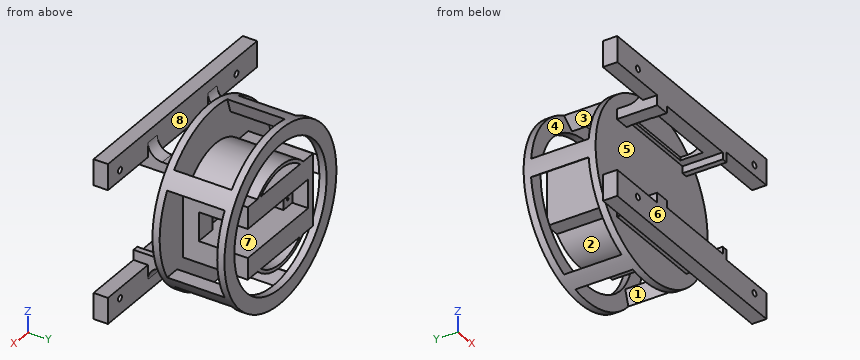
```python
from build123d import *

# Parameters (mm, degrees)
ESQUISSE1_W                  = 70
ESQUISSE1_H                  = 50
BOSS_EXTRU_1_DEPTH           = 50
ESQUISSE2_W                  = 40.5
ESQUISSE2_H                  = 20
ENL_V_MAT_EXTRU_1_DEPTH      = 38
ESQUISSE3_W                  = 9.502474521
ESQUISSE3_H                  = 20
ENL_V_MAT_EXTRU_2_DEPTH      = 11
ESQUISSE4_R                  = 60.076490873
ESQUISSE4_R_2                = 49.5
BOSS_EXTRU_2_DEPTH           = 50
ESQUISSE5_W                  = 60
ESQUISSE5_H                  = 40
ENL_V_MAT_EXTRU_3_DEPTH      = 24
R_P_TITION_START             = -20
R_P_TITION_CIRCULAIRE1_DEPTH = 40
ESQUISSE12_W                 = 74.3
ESQUISSE12_H                 = 74.3
BOSS_EXTRU_7_DEPTH           = 28
ESQUISSE13_W                 = 160
ESQUISSE13_H                 = 18
BOSS_EXTRU_8_DEPTH           = 10
ESQUISSE15_R                 = 60.076490873
BOSS_EXTRU_9_DEPTH           = 5
ESQUISSE16_W                 = 60
ESQUISSE16_H                 = 70
ENL_V_MAT_EXTRU_4_DEPTH      = 28
ENL_V_MAT_EXTRU_5_REACH      = 156.276
ESQUISSE17_W                 = 60.3
ESQUISSE17_H                 = 28
ENL_V_MAT_EXTRU_6_REACH      = 138.609
ESQUISSE18_W                 = 54.3
ESQUISSE18_H                 = 15.510808694
TROU_TARAUD_M5X0_82_D        = 4.2
TROU_TARAUD_M5X0_82_DEPTH    = 54.927
TROU_TARAUD_M5X0_82_TIP      = 1.2618073
TROU_TARAUD_M5X0_83_D        = 4.2
TROU_TARAUD_M5X0_83_DEPTH    = 54.927
TROU_TARAUD_M5X0_83_TIP      = 1.2618073
CONG_1_R                     = 10
ESQUISSE25_W                 = 16.470730929
ESQUISSE25_H                 = 20
ENL_V_MAT_EXTRU_7_DEPTH      = 34
TROU_TARAUD_M2X0_41_D        = 1.6
TROU_TARAUD_M2X0_41_DEPTH    = 15
TROU_TARAUD_M2X0_41_TIP      = 0.480688495


# Read off the part's stored shape, not the designer's step: Répétition circulaire1
with BuildPart() as part:
    # Esquisse1 → Boss.-Extru.1 (new body)
    with BuildSketch(Plane.XY):
        Rectangle(ESQUISSE1_W, ESQUISSE1_H)
    extrude(amount=BOSS_EXTRU_1_DEPTH)

    # Esquisse2 → Enlèv. mat.-Extru.1 (cut)
    with BuildSketch(Plane(origin=(0, 25, 0), x_dir=(1, 0, 0), z_dir=(0, 1, 0))):
        with Locations((0, -25)):
            Rectangle(ESQUISSE2_W, ESQUISSE2_H)
    extrude(amount=-ENL_V_MAT_EXTRU_1_DEPTH, mode=Mode.SUBTRACT)

    # Esquisse3 → Enlèv. mat.-Extru.2 (cut)
    with BuildSketch(Plane(origin=(0, 25, 0), x_dir=(1, 0, 0), z_dir=(0, 1, 0))):
        with Locations((25.001237261, -25)):
            Rectangle(ESQUISSE3_W, ESQUISSE3_H)
        with Locations((-25.001237261, -25)):
            Rectangle(ESQUISSE3_W, ESQUISSE3_H)
    extrude(amount=-ENL_V_MAT_EXTRU_2_DEPTH, mode=Mode.SUBTRACT)

    # Esquisse4 → Boss.-Extru.2 (add)
    # profile 1 of 7: a face of its own
    with BuildSketch(Plane(origin=(0, 25, 0), x_dir=(1, 0, 0), z_dir=(0, 1, 0))):
        with Locations(Location((0, -25.176679726, 0), (0, 0, 270))):
            Circle(ESQUISSE4_R)
        with Locations(Location((0, -25.176679726, 0), (0, 0, 270))):
            Circle(ESQUISSE4_R_2, mode=Mode.SUBTRACT)
    # profile 2 of 7: a face of its own
    with BuildSketch(Plane(origin=(0, 25, 0), x_dir=(1, 0, 0), z_dir=(0, 1, 0))):
        with BuildLine():
            ThreePointArc((24.673928965, -50), (32.315534297, -38.619381951), (35, -25.176679726))
            ThreePointArc((35, -25.176679726), (32.217729855, -11.501231543), (24.313263828, 0))
            Line((24.313263828, 0), (20.744399349, 0))
            ThreePointArc((20.744399349, 0), (29.503552635, -11.257782921), (32.622006474, -25.176679726))
            ThreePointArc((32.622006474, -25.176679726), (29.619854452, -38.846336948), (21.16596506, -50))
            Line((21.16596506, -50), (24.673928965, -50))
        make_face()
    # profile 3 of 7: a face of its own
    with BuildSketch(Plane(origin=(0, 25, 0), x_dir=(1, 0, 0), z_dir=(0, 1, 0))):
        with BuildLine():
            Line((-20.744399349, 0), (-24.313263828, 0))
            ThreePointArc((-24.313263828, 0), (-34.99908948, -24.924220698), (-24.673928965, -50))
            Line((-24.673928965, -50), (-21.16596506, -50))
            ThreePointArc((-21.16596506, -50), (-32.620847034, -24.901643114), (-20.744399349, 0))
        make_face()
    # profile 4 of 7: a face of its own
    with BuildSketch(Plane(origin=(0, 25, 0), x_dir=(1, 0, 0), z_dir=(0, 1, 0))):
        with BuildLine():
            Line((20.744399349, 0), (24.313263828, 0))
            ThreePointArc((24.313263828, 0), (0, 9.823320274), (-24.313263828, 0))
            Line((-24.313263828, 0), (-20.744399349, 0))
            ThreePointArc((-20.744399349, 0), (0, 7.445326748), (20.744399349, 0))
        make_face()
    # profile 5 of 7: a face of its own
    with BuildSketch(Plane(origin=(0, 25, 0), x_dir=(1, 0, 0), z_dir=(0, 1, 0))):
        with BuildLine():
            ThreePointArc((24.673928965, -50), (32.315534297, -38.619381951), (35, -25.176679726))
            ThreePointArc((35, -25.176679726), (32.217729855, -11.501231543), (24.313263828, 0))
            Line((24.313263828, 0), (20.744399349, 0))
            ThreePointArc((20.744399349, 0), (29.503552635, -11.257782921), (32.622006474, -25.176679726))
            ThreePointArc((32.622006474, -25.176679726), (29.619854452, -38.846336948), (21.16596506, -50))
            Line((21.16596506, -50), (24.673928965, -50))
        make_face()
    # profile 6 of 7: a face of its own
    with BuildSketch(Plane(origin=(0, 25, 0), x_dir=(1, 0, 0), z_dir=(0, 1, 0))):
        with BuildLine():
            Line((-20.744399349, 0), (-24.313263828, 0))
            ThreePointArc((-24.313263828, 0), (-34.99908948, -24.924220698), (-24.673928965, -50))
            Line((-24.673928965, -50), (-21.16596506, -50))
            ThreePointArc((-21.16596506, -50), (-32.620847034, -24.901643114), (-20.744399349, 0))
        make_face()
    # profile 7 of 7: a face of its own
    with BuildSketch(Plane(origin=(0, 25, 0), x_dir=(1, 0, 0), z_dir=(0, 1, 0))):
        with BuildLine():
            ThreePointArc((-24.673928965, -50), (0, -60.176679726), (24.673928965, -50))
            Line((24.673928965, -50), (21.16596506, -50))
            ThreePointArc((21.16596506, -50), (0, -57.798686199), (-21.16596506, -50))
            Line((-21.16596506, -50), (-24.673928965, -50))
        make_face()
    extrude(amount=-BOSS_EXTRU_2_DEPTH)


with BuildPart() as boss_extru_2_piece_1:
    # of the separate pieces the step leaves, piece 1, a body of its own (boss_extru_2_pieces)
    add(part.part.solids().sort_by_distance((0, 25, 85.253170599))[0])

    # Esquisse5 → Enlèv. mat.-Extru.3 (cut)
    with BuildSketch(Plane(origin=(60.076490873, 0, 0), x_dir=(0, 0, -1), z_dir=(1, 0, 0))):
        with Locations((-25.176679726, 0)):
            Rectangle(ESQUISSE5_W, ESQUISSE5_H)
    extrude(amount=-ENL_V_MAT_EXTRU_3_DEPTH, mode=Mode.SUBTRACT)

    # Répétition circulaire1 outline → Répétition circulaire1 (cut)
    with BuildSketch(Plane(origin=(0, 0, 0), x_dir=(1, 0, 0), z_dir=(0, 1, 0)).offset(R_P_TITION_START)):
        with BuildLine():
            Line((39.373214245, 4.823320274), (41.291457614, 4.823320274))
            Line((41.291457614, 4.823320274), (44.615977372, 15.055140003))
            ThreePointArc((44.615977372, 15.055140003), (18.564656642, 31.959458395), (-12.447413605, 33.596159666))
            Line((-12.447413605, 33.596159666), (-15.771933364, 23.364339937))
            Line((-15.771933364, 23.364339937), (-24.475639087, 29.687952296))
            ThreePointArc((-24.475639087, 29.687952296), (-48.602902078, 10.135395619), (-59.742754225, -18.853067366))
            Line((-59.742754225, -18.853067366), (-51.039048501, -25.176679726))
            Line((-51.039048501, -25.176679726), (-59.742754225, -31.500292085))
            ThreePointArc((-59.742754225, -31.500292085), (-48.602902079, -60.488755071), (-24.475639087, -80.041311748))
            Line((-24.475639087, -80.041311748), (-15.771933364, -73.717699388))
            Line((-15.771933364, -73.717699388), (-12.447413605, -83.949519118))
            ThreePointArc((-12.447413605, -83.949519118), (18.564656643, -82.312817847), (44.615977373, -65.408499455))
            Line((44.615977373, -65.408499455), (41.291457614, -55.176679726))
            Line((41.291457614, -55.176679726), (39.373214245, -55.176679726))
            ThreePointArc((39.373214245, -55.176679726), (-49.5, -25.176679726), (39.373214245, 4.823320274))
        make_face()
    extrude(amount=R_P_TITION_CIRCULAIRE1_DEPTH, mode=Mode.SUBTRACT)



with BuildPart() as boss_extru_2_piece_2:
    # of the separate pieces the step leaves, piece 2, a body of its own (boss_extru_2_pieces)
    add(part.part.solids().sort_by_distance((-35, 25, 0))[0])


with BuildPart() as boss_extru_2_piece_1_1:
    add(boss_extru_2_piece_1.part)

    add(boss_extru_2_piece_2.part)  # Boss.-Extru.7 merges Boss.-Extru.2 piece 2
    # Esquisse12 → Boss.-Extru.7 (add)
    with BuildSketch(Plane.XZ.offset(25)):
        with Locations((0, 25.176679726)):
            Rectangle(ESQUISSE12_W, ESQUISSE12_H)
    extrude(amount=BOSS_EXTRU_7_DEPTH)

    # Esquisse13 → Boss.-Extru.8 (add)
    with BuildSketch(Plane.XZ.offset(53)):
        with Locations((0, 71.326679726)):
            Rectangle(ESQUISSE13_W, ESQUISSE13_H)
        with Locations((0, -20.973320274)):
            Rectangle(ESQUISSE13_W, ESQUISSE13_H)
    extrude(amount=-BOSS_EXTRU_8_DEPTH)

    # Esquisse15 → Boss.-Extru.9 (add)
    with BuildSketch(Plane(origin=(0, -20, 0), x_dir=(1, 0, 0), z_dir=(0, 1, 0))):
        with Locations(Location((0, -25.176679726, 0), (0, 0, 270))):
            Circle(ESQUISSE15_R)
    extrude(amount=-BOSS_EXTRU_9_DEPTH)

    # Esquisse16 → Enlèv. mat.-Extru.4 (cut)
    with BuildSketch(Plane.XZ.offset(53)):
        with Locations((3.15, 25.176679726)):
            Rectangle(ESQUISSE16_W, ESQUISSE16_H)
    extrude(amount=-ENL_V_MAT_EXTRU_4_DEPTH, mode=Mode.SUBTRACT)

    # Enlèv. mat.-Extru.5: up to this face of the body (flat: up to its plane)
    enl_v_mat_extru_5_end = Plane(boss_extru_2_piece_1_1.part.faces().sort_by_distance((-37.15, -39, 25.176679726))[0])
    # Esquisse17 → Enlèv. mat.-Extru.5 (cut, up to the picked face)
    with BuildSketch(Plane(origin=(37.15, 0, 0), x_dir=(0, 0, -1), z_dir=(1, 0, 0)), mode=Mode.PRIVATE) as enl_v_mat_extru_5_sk1:
        with Locations((-25.176679726, -39)):
            Rectangle(ESQUISSE17_W, ESQUISSE17_H)
    enl_v_mat_extru_5_tool1 = split(extrude(enl_v_mat_extru_5_sk1.sketch, amount=-ENL_V_MAT_EXTRU_5_REACH, mode=Mode.PRIVATE), bisect_by=enl_v_mat_extru_5_end, keep=Keep.BOTH, mode=Mode.PRIVATE)
    add(enl_v_mat_extru_5_tool1.solids().sort_by(Axis((37.15, -39, 25.17668), (-1, 0, 0)))[0], mode=Mode.SUBTRACT)

    # Enlèv. mat.-Extru.6: up to this face of the body (flat: up to its plane)
    enl_v_mat_extru_6_end = Plane(boss_extru_2_piece_1_1.part.faces().sort_by_distance((0, -34, -11.973320274))[0])
    # Esquisse18 → Enlèv. mat.-Extru.6 (cut, up to the picked face)
    with BuildSketch(Plane.XY.offset(62.326679726), mode=Mode.PRIVATE) as enl_v_mat_extru_6_sk1:
        with Locations((0, -35.244595653)):
            Rectangle(ESQUISSE18_W, ESQUISSE18_H)
    enl_v_mat_extru_6_tool1 = split(extrude(enl_v_mat_extru_6_sk1.sketch, amount=-ENL_V_MAT_EXTRU_6_REACH, mode=Mode.PRIVATE), bisect_by=enl_v_mat_extru_6_end, keep=Keep.BOTH, mode=Mode.PRIVATE)
    add(enl_v_mat_extru_6_tool1.solids().sort_by(Axis((0, -35.244596, 62.32668), (0, 0, -1)))[0], mode=Mode.SUBTRACT)

    # Trou taraudé M5x0.82
    with Locations(Plane(origin=(-57.931903984, -53, -18.999181229), x_dir=(0, 0, -1), z_dir=(0, -1, 0))):
        with Locations((0, 0), (-88.38422, 0.087735642)):
            Hole(TROU_TARAUD_M5X0_82_D / 2, depth=TROU_TARAUD_M5X0_82_DEPTH)
            with Locations((0, 0, -(TROU_TARAUD_M5X0_82_DEPTH + TROU_TARAUD_M5X0_82_TIP / 2))):  # 118° drill point
                Cone(0, TROU_TARAUD_M5X0_82_D / 2, TROU_TARAUD_M5X0_82_TIP, mode=Mode.SUBTRACT)

    # Trou taraudé M5x0.83
    with Locations(Plane(origin=(67.121659864, -53, 69.376817601), x_dir=(0, 0, -1), z_dir=(0, -1, 0))):
        with Locations((0, 0), (88.384296015, 0.049521474)):
            Hole(TROU_TARAUD_M5X0_83_D / 2, depth=TROU_TARAUD_M5X0_83_DEPTH)
            with Locations((0, 0, -(TROU_TARAUD_M5X0_83_DEPTH + TROU_TARAUD_M5X0_83_TIP / 2))):  # 118° drill point
                Cone(0, TROU_TARAUD_M5X0_83_D / 2, TROU_TARAUD_M5X0_83_TIP, mode=Mode.SUBTRACT)

    # Congé1
    cong_1_edges = [boss_extru_2_piece_1_1.edges().sort_by_distance(p)[0] for p in [
        (-32.15, -43, 62.326679726),
        (32.15, -43, -11.973320274),
        (32.15, -43, 62.326679726),
        (-32.15, -43, -11.973320274),
    ]]
    fillet(cong_1_edges, radius=CONG_1_R)

    # Esquisse25 → Enlèv. mat.-Extru.7 (cut)
    with BuildSketch(Plane(origin=(0, 25, 0), x_dir=(1, 0, 0), z_dir=(0, 1, 0))):
        with Locations((26.764634536, -25)):
            Rectangle(ESQUISSE25_W, ESQUISSE25_H)
    extrude(amount=-ENL_V_MAT_EXTRU_7_DEPTH, mode=Mode.SUBTRACT)

    # Trou taraudé M2x0.41
    with Locations(Plane(origin=(-24.71, 14, 20.075), x_dir=(0, 0, 1), z_dir=(0, 1, 0))):
        with Locations((0, 0), (9.85, 0)):
            Hole(TROU_TARAUD_M2X0_41_D / 2, depth=TROU_TARAUD_M2X0_41_DEPTH)
            with Locations((0, 0, -(TROU_TARAUD_M2X0_41_DEPTH + TROU_TARAUD_M2X0_41_TIP / 2))):  # 118° drill point
                Cone(0, TROU_TARAUD_M2X0_41_D / 2, TROU_TARAUD_M2X0_41_TIP, mode=Mode.SUBTRACT)


solid = boss_extru_2_piece_1_1.part
```
Source: CAD feature listing. Evaluate the final solid. Frame: model axes, mm. Face numbers are marked on the shaded views. A direction names the side the tool comes from. Round coordinates to 2 decimals unless told otherwise and drop trailing zeros. Loops run counter-clockwise (first coordinate to the right, second up) from the corner with the lowest first, then second, coordinate; pieces in that order, holes last.
1. Access query for the marked faces 1, 2, 3 and 4. Directions: +Z, -Z, +X, -X, +Y, -Y. A direction counts if a zero-diameter tool reaches every point of the face in a straight line with its end or side. Return the directions, or none.
2. Ray query, L1, parallel to Z at x = -24.71, y = 3.75 (3 decimals); L2, parallel to Z at x = -8.5, y = -19; L3, parallel to X at y = -36, z = 62. Return the intervals inside material, ascending.
3. Mould query, pull axis Y, two halves, no side actions, for the marked faces 5, 6, 7 and 8. Classes: released by +Y, released by -Y, zero draft, split by the parting line, or undercut.
4. Section query C-C on z = 2.5. Output: boundary loops of the cut face in (x, y).
5. Contact query for flat-ended pins moving along their axis: pin 1 (1 mm diameter, centred on x = -53, z = 46, fed in from -Y); pin 2 (8 mm diameter, centred on x = -49.5, y = -47.5, fed in from +Z); pin 3 (6 mm diameter, centred on x = -1.5, z = 26.5, fed in from +Y); pin 4 (5 mm diameter, centred on y = -37, z = 67.5, fed in from +X). Output: stop coordinate, or through.
6. Section query A-A on y = 2. Give the number of separate pieces and of enclosed holes in the cut face, and give its area (3 significant figures).
7. Section query B-B on y = -45. Output: boundary loops of the cut face in (x, z).
Answers below:
1. face 1: -Z
1. face 2: +Y
1. face 3: -X
1. face 4: none
2. L1: z = 0 to 19.275, 20.875 to 29.125, 30.725 to 50
2. L2: z = -8.78 to -6.32, 0 to 50, 56.67 to 59.13
2. L3: x = -37.15 to -27.15, 27.15 to 37.15
3. face 5: undercut
3. face 6: released by -Y
3. face 7: zero draft
3. face 8: undercut
4. outline: (-55.63, -25) - (55.63, -25) - (55.63, -20) - (35, -20) - (35, 25) - (-35, 25) - (-35, -20) - (-55.63, -20) - close; (-55.63, 20) - (-44, 20) - (-44, 25) - (-55.63, 25) - close; (44, 20) - (55.63, 20) - (55.63, 25) - (44, 25) - close
5. pin 1: stops at y = -25
5. pin 2: stops at z = 80.33
5. pin 3: stops at y = -13
5. pin 4: passes through
6. separate pieces: 6
6. enclosed holes: 4
6. area: 2,920 mm2
7. outline: (-80, -29.97) - (80, -29.97) - (80, -11.97) - (37.15, -11.97) - (37.15, -4.97) - (33.15, -4.97) - (33.15, -9.82) - (-26.85, -9.82) - (-26.85, -4.97) - (-37.15, -4.97) - (-37.15, -11.97) - (-80, -11.97) - close; (-80, 62.33) - (-37.15, 62.33) - (-37.15, 55.33) - (-26.85, 55.33) - (-26.85, 60.18) - (33.15, 60.18) - (33.15, 55.33) - (37.15, 55.33) - (37.15, 62.33) - (80, 62.33) - (80, 80.33) - (-80, 80.33) - close; hole circle Ø4.2 at (-57.93, -19); hole circle Ø4.2 at (-57.84, 69.39); hole circle Ø4.2 at (67.12, 69.38); hole circle Ø4.2 at (67.17, -19.01)
